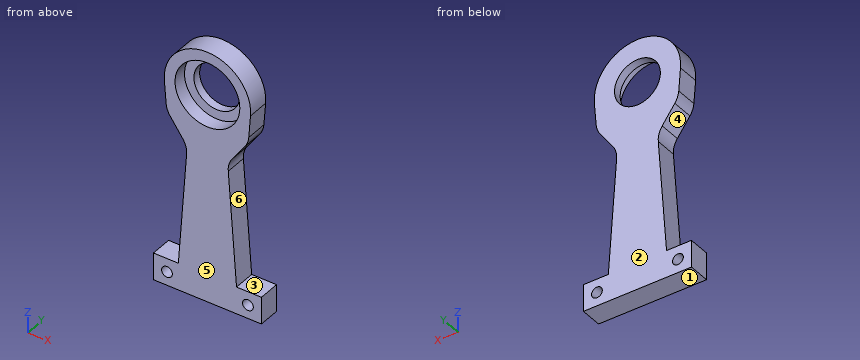
```python
from build123d import *

# Parameters (mm, degrees)
F0_R     = 12
F1_DEPTH = 8
F3_DEPTH = 25
F4_R     = 8
F5_R     = 12
F5_R_2   = 8.5
F6_DEPTH = 3
F7_R     = 2
F8_DEPTH = 25


with BuildPart() as f1:
    # F0 (on Front) → F1 (new body)
    with BuildSketch(Plane.XZ):
        with BuildLine():
            Line((10.7804718609, -67.5), (15.9514905981, -1.2449689551))
            ThreePointArc((15.9514905981, -1.2449689551), (0, 16), (-15.9514905981, -1.2449689551))
            Line((-15.9514905981, -1.2449689551), (-10.7804718609, -67.5))
            Line((-10.7804718609, -67.5), (-20, -67.5))
            Line((-20, -67.5), (-20, -77.5))
            Line((-20, -77.5), (-10, -77.5))
            Line((-10, -77.5), (10, -77.5))
            Line((10, -77.5), (20, -77.5))
            Line((20, -77.5), (20, -67.5))
            Line((20, -67.5), (10.7804718609, -67.5))
        make_face()
        Circle(F0_R, mode=Mode.SUBTRACT)
    extrude(amount=F1_DEPTH)

    # F2 (on face) → F3 (cut)
    with BuildSketch(Plane(origin=(0, 0, 0), x_dir=(-1, 0, 0), z_dir=(0, 1, 0))):
        Polygon((-7.5, -22.5), (-15.1268365117, -11.8110652832), (-10.7804718609, -67.5), align=None)
        Polygon((10.7804718609, -67.5), (15.1268365117, -11.8110652832), (7.5, -22.5), align=None)
    extrude(amount=-F3_DEPTH, mode=Mode.SUBTRACT)

    # F4
    f4_edges = [f1.edges().sort_by_distance(p)[0] for p in [
        (-7.5, -4, -22.5),
        (-15.126837, -4, -11.811065),
        (15.126837, -4, -11.811065),
        (7.5, -4, -22.5),
    ]]
    fillet(f4_edges, radius=F4_R)

    # F5 (on face) → F6 (join)
    with BuildSketch(Plane(origin=(0, 0, 0), x_dir=(-1, 0, 0), z_dir=(0, 1, 0))):
        with BuildLine():
            Line((20, -67.5), (10.7804718609, -67.5))
            Line((10.7804718609, -67.5), (7.7098565421, -25.3787152568))
            ThreePointArc((7.7098565421, -25.3787152568), (7.9860060263, -22.6363328806), (9.1764777393, -20.150433298))
            Line((9.1764777393, -20.150433298), (13.8361972063, -13.6198832981))
            ThreePointArc((13.8361972063, -13.6198832981), (14.8422105338, -11.7075498191), (15.2997366254, -9.5957373215))
            Line((15.2997366254, -9.5957373215), (15.9514905981, -1.2449689551))
            ThreePointArc((15.9514905981, -1.2449689551), (0, 16), (-15.9514905981, -1.2449689551))
            Line((-15.9514905981, -1.2449689551), (-15.2997366254, -9.5957373215))
            ThreePointArc((-15.2997366254, -9.5957373215), (-14.8422105338, -11.7075498191), (-13.8361972063, -13.6198832981))
            Line((-13.8361972063, -13.6198832981), (-9.1764777393, -20.150433298))
            ThreePointArc((-9.1764777393, -20.150433298), (-7.9860060263, -22.6363328806), (-7.7098565421, -25.3787152568))
            Line((-7.7098565421, -25.3787152568), (-10.7804718609, -67.5))
            Line((-10.7804718609, -67.5), (-20, -67.5))
            Line((-20, -67.5), (-20, -77.5))
            Line((-20, -77.5), (20, -77.5))
            Line((20, -77.5), (20, -67.5))
        make_face()
        Circle(F5_R, mode=Mode.SUBTRACT)
        Circle(F5_R)
        Circle(F5_R_2, mode=Mode.SUBTRACT)
    extrude(amount=-F6_DEPTH)

    # F7 (on face) → F8 (cut)
    with BuildSketch(Plane.XZ.offset(8)):
        with Locations((-15, -72.5)):
            Circle(F7_R)
        with Locations((15, -72.5)):
            Circle(F7_R)
    extrude(amount=-F8_DEPTH, mode=Mode.SUBTRACT)


solid = f1.part
```
Geometry: final body of the model. Coordinates: model frame, mm. Face numbers are marked on the shaded views. A direction names the side the tool comes from. Round coordinates to 2 decimals unless told otherwise and drop trailing zeros. Order: outer loops, then holes, each group sorted by start corner. A loop starts at its lowest first (then second) coordinate and runs counter-clockwise, first axis right, second up. Notation, with made-up numbers: (-22.75, -26) - (8.25, -26) arc R15 cw to (8.25, -14) - close; hole circle Ø5 at (68.5, 38.5). An arc over 180 degrees is marked (long way). Write item = value, one per line. Start each with the question number.
Q1. Cut plane D-D on z = -34.5. Return the cut outline in (x, y), and give its area (3 significant figures).
Q2. Pull-direction query (Z, two-part tool) for the marked faces 1, 2 and 3; classes: +Z half, -Z half, draft (parallel to the pull), parting line (faces both ways), or undercut.
Q3. Ray query, line 1 (X direction, y = -6.5, z = 0); line 2 (X direction, y = -3.75, z = -71); line 3 (Z direction, x = -3, y = -4.75). Return the intervals inside material, ascending. Write a range as from..to.
Q4. Cut plane A-A on x = 0. Return the cut outline in (y, z).
Q5. Pin query (flat end, axial travel): pin 1 (4 mm diameter, centred on x = -4.5, z = -7.5, fed in from -Y); pin 2 (4 mm diameter, centred on x = -15, y = -3.5, fed in from +Z); pin 3 (1 mm diameter, centred on x = 10, y = -7, fed in from +Z). Return the tip coordinate at first contact, or that it passes through.
Q6. Access query for the marked faces 4, 5 and 6. Directions: +Z, -Z, +X, -X, +Y, -Y. A direction counts if a zero-diameter tool reaches every point of the face in a straight line with its end or side. Return the directions, or none.
Q7. Cut plane B-B on z = 0. Return the cut outline in (x, y), and give its area (3 significant figures).
Q8. Cut plane C-C on y = -6.5. Return the cut outline in (x, z), and give its area (3 significant figures).
Outcome:
q1.outline = (-8.37, -8) - (8.37, -8) - (8.37, 0) - (-8.37, 0) - close
q1.area = 134 mm^2
q2.face_1 = -Z half
q2.face_2 = draft
q2.face_3 = undercut
q3.line_1 = -16..-12, 12..16
q3.line_2 = -20..-16.32, -13.68..13.68, 16.32..20
q3.line_3 = -77.5..-11.62, 11.62..15.72
q4.outline = (-8, -77.5) - (0, -77.5) - (0, -8.5) - (-3, -8.5) - (-3, -12) - (-8, -12) - close; (-8, 12) - (-3, 12) - (-3, 8.5) - (0, 8.5) - (0, 16) - (-8, 16) - close
q5.pin_1 = -3
q5.pin_2 = 9.33
q5.pin_3 = 12.87
q6.face_4 = -X, +Y, -Y
q6.face_5 = +Z, -Z, +X, -X, -Y
q6.face_6 = +X, +Y, -Y
q7.outline = (-16, -8) - (-12, -8) - (-12, -3) - (-8.5, -3) - (-8.5, 0) - (-16, 0) - close; (8.5, -3) - (12, -3) - (12, -8) - (16, -8) - (16, 0) - (8.5, 0) - close
q7.area = 85.0 mm^2
q8.outline = (-20, -77.5) - (20, -77.5) - (20, -67.5) - (10.78, -67.5) - (7.71, -25.38) arc R8 cw to (9.18, -20.15) - (13.84, -13.62) arc R8 ccw to (15.3, -9.6) - (15.95, -1.24) arc R16 ccw (long way) to (-15.95, -1.24) - (-15.3, -9.6) arc R8 ccw to (-13.84, -13.62) - (-9.18, -20.15) arc R8 cw to (-7.71, -25.38) - (-10.78, -67.5) - (-20, -67.5) - close; hole circle Ø4 at (-15, -72.5); hole circle Ø24 at (0, 0); hole circle Ø4 at (15, -72.5)
q8.area = 1,760 mm^2
